Here's how the part is built. I have some questions about the finished solid (model axes, mm). A direction names the side the tool comes from. Give positions to 0.01 mm unless a question says otherwise; leave off trailing zeros. Order: outer loops, then holes, each group sorted by start corner. A loop starts at its lowest first (then second) coordinate and runs counter-clockwise, first axis right, second up.
Autodesk Inventor part; units mm, degrees
ref_plane "YZ Plane" through (0, 0, 0) normal (1, 0, 0) x (0, 1, 0)
ref_plane "XZ Plane" through (0, 0, 0) normal (0, 1, 0) x (-1, 0, 0)
ref_plane "XY Plane" through (0, 0, 0) normal (0, 0, 1) x (1, 0, 0)
sketch "Sketch1" plane through (0, 0, 0) normal (0, 1, 0) x (-1, 0, 0)
  line L0 (0, 0) -> (-20, 0)
  line L1 (-20, 0) -> (-20, -3)
  line L2 (-20, -3) -> (0, -3)
  line L3 (0, -3) -> (0, 0)
  line L4 (3, -6) -> (-23, -6)
  line L5 (-23, -6) -> (-23, 3)
  line L6 (-23, 3) -> (3, 3)
  line L7 (3, 3) -> (3, -6)
  line L8 (-30, -6) -> (-30, 3)
  line L9 (10, 3) -> (10, -6)
  line L10 (3, -6) -> (10, -6)
  line L11 (3, 3) -> (10, 3)
  line L12 (-23, 3) -> (-30, 3)
  line L13 (-23, -6) -> (-30, -6)
  line L14 (10, -6) -> (13, -6)
  line L15 (13, -6) -> (13, 3)
  line L16 (13, 3) -> (10, 3)
  line L17 (-30, 3) -> (-33, 3)
  line L18 (-33, 3) -> (-33, -6)
  line L19 (-33, -6) -> (-30, -6)
  line L20 (0, 0) -> (10, 0)
  line L21 (0, -3) -> (10, -3)
  line L22 (-20, 0) -> (-30, 0)
  line L23 (-20, -3) -> (-30, -3)
  dimension "d0" = 20
  dimension "d1" = 3
  dimension "d2" = 3
  dimension "d6" = 40
  dimension "d7" = 3
  dimension "d8" = 3
extrude "Extrusion1" add sketch "Sketch1" against normal blind 3 contours L20 L7 L21 L3 | L0 L22 L5 L6 L7 L20 | L1 L23 L5 L22 | L21 L7 L4 L5 L23 L2 | L20 L9 L21 L7 | L7 L11 L9 L20 | L22 L8 L12 L5 | L5 L23 L8 L22 | L21 L9 L10 L7 | L9 L16 L15 L14 | L5 L13 L8 L23 | L8 L19 L18 L17
extrude "Extrusion2" add sketch "Sketch1" along normal blind 40 contours L0 L22 L5 L6 L7 L20 | L21 L7 L4 L5 L23 L2 | L7 L11 L9 L20 | L22 L8 L12 L5 | L21 L9 L10 L7 | L9 L16 L15 L14 | L5 L13 L8 L23 | L8 L19 L18 L17
sketch "Sketch2" plane through (0, 40, 0) normal (0, 1, 0) x (1, 0, 0)
  line L0 (33, 6) -> (-13, 6)
  line L1 (-13, 6) -> (-13, -3)
  line L2 (-13, -3) -> (33, -3)
  line L3 (33, -3) -> (33, 6)
  line L4 (-10, 3) -> (30, 3)
  line L5 (30, 3) -> (30, 0)
  line L6 (30, 0) -> (-10, 0)
  line L7 (-10, 0) -> (-10, 3)
  point P0 (0, 0)
extrude "Extrusion3" add sketch "Sketch2" along normal blind 3 contours L3 L2 L1 L0 | L4 L5 L6 L7
sketch "Sketch3" plane through (-13, -3, 3) normal (0, 0, 1) x (1, 0, 0)
  line L0 (7, 43) -> (39, 43)
  line L1 (43, 39) -> (43, 7)
  line L2 (39, 3) -> (7, 3)
  line L3 (3, 7) -> (3, 39)
  line L4 (0, 46) -> (0, 0)
  line L5 (46, 0) -> (0, 0)
  line L6 (46, 0) -> (46, 46)
  line L7 (0, 46) -> (46, 46)
  arc A0 (7, 43) -> (3, 39) centre (7, 39) ccw
  arc A1 (43, 39) -> (39, 43) centre (39, 39) ccw
  arc A2 (39, 3) -> (43, 7) centre (39, 7) ccw
  arc A3 (3, 7) -> (7, 3) centre (7, 7) ccw
  line L8 (43, 3) -> (33, 3)
  line L9 (43, 3) -> (39, 3)
  line L10 (43, 3) -> (43, 43)
  line L11 (43, 3) -> (43, 7)
  point P0 (13, 3)
  point P1 (3, 43)
  point P2 (3, 3)
  dimension "d13" = 40
  dimension "d14" = 40
  dimension "d15" = 3
  dimension "d16" = 3
  dimension "d21" = 4
extrude "Extrusion4" cut sketch "Sketch3" against normal blind 3 contours L0 A1 L1 A2 L2 A3 L3 A0
extrude "Extrusion6" add sketch "Sketch3" against normal blind 8 contours L10 L8 A2 | L7 L6 L5 L4
extrude "Extrusion7" add sketch "Sketch3" along normal blind 10.5 contours L10 L8 A2 | L7 L6 L5 L4
extrude "Extrusion8" cut sketch "Sketch1" against normal blind 10.5 contours L3 L2 L1 L0
fillet "Fillet1" radius 5 4 edges at (-13, 43, 3.75) (33, 43, 3.75) (-13, -3, 3.75) (33, -3, 3.75)
sketch "Sketch4" plane through (-13, -3, 13.5) normal (0, 0, 1) x (1, 0, 0)
  arc A0 (41, 0) -> (46, 5) centre (41, 5) ccw
  line L0 (46, 5) -> (46, 41)
  arc A1 (46, 41) -> (41, 46) centre (41, 41) ccw
  line L1 (41, 46) -> (5, 46)
  arc A2 (5, 46) -> (0, 41) centre (5, 41) ccw
  line L2 (0, 41) -> (0, 5)
  arc A3 (0, 5) -> (5, 0) centre (5, 5) ccw
  line L3 (5, 0) -> (41, 0)
  line L4 (7, 43) -> (39, 43)
  arc A4 (43, 39) -> (39, 43) centre (39, 39) ccw
  line L5 (43, 39) -> (43, 7)
  arc A5 (39, 3) -> (43, 7) centre (39, 7) ccw
  line L6 (39, 3) -> (7, 3)
  arc A6 (3, 7) -> (7, 3) centre (7, 7) ccw
  line L7 (3, 7) -> (3, 39)
  arc A7 (7, 43) -> (3, 39) centre (7, 39) ccw
  arc A8 (0, 5) -> (5, 0) centre (5, 5) ccw
  line L8 (0, 5) -> (-2.5, 5)
  line L9 (-7.5, 10) -> (-7.5, 10)
  line L10 (-2.5, 15) -> (0, 15)
  arc A9 (-2.5, 15) -> (-7.5, 10) centre (-2.5, 10) ccw
  arc A10 (-7.5, 10) -> (-2.5, 5) centre (-2.5, 10) ccw
  line L11 (46, 5) -> (48.5, 5)
  line L12 (53.5, 10) -> (53.5, 10)
  line L13 (48.5, 15) -> (46, 15)
  line L14 (46, 15) -> (46, 5)
  circle A11 centre (48.5, 10) radius 2.5
  arc A12 (53.5, 10) -> (48.5, 15) centre (48.5, 10) ccw
  arc A13 (48.5, 5) -> (53.5, 10) centre (48.5, 10) ccw
  circle A14 centre (-2.5, 10) radius 2.5
  point P0 (13, 3)
  point P1 (-7.5, 5)
  point P2 (-7.5, 15)
  point P3 (-7.5, 10)
  point P4 (53.5, 15)
  point P5 (53.5, 5)
  point P6 (53.5, 10)
  point P7 (46, 10)
  point P8 (-7.5, 10)
  point P9 (0, 10)
  dimension "d29" = 7.5
  dimension "d30" = 10
  dimension "d33" = 5
  dimension "d34" = 7.5
  dimension "d35" = 10
  dimension "d36" = 5
  dimension "d37" = 5
  dimension "d38" = 5
  dimension "d41" = 5
extrude "Extrusion9" add sketch "Sketch4" against normal blind 10 contours L0 L13 A12 A13 L11 | L8 A10 A9 L10 L2
fillet "Fillet2" radius 2 3 edges at (-10, 20, -3) (10, 40, -3) (30, 20, -3)
fillet "Fillet4" radius 2.5 6 edges at (34.25, 2, 3.5) (34.25, 12, 3.5) (40.5, 7, 3.5) (-14.25, 12, 3.5) (-14.25, 2, 3.5) (-20.5, 7, 3.5)
properties part number "FANHOLDER_3DPrint"
Q1. If we section it at B-B on z = 10.75: List the corners of the cut face in (x, y) for me.
Filled sheet:
outline: (-15.5, 2) - (-13, 2) arc R5 ccw to (-8, -3) - (28, -3) arc R5 ccw to (33, 2) - (35.5, 2) arc R5 ccw to (35.5, 12) - (33, 12) - (33, 38) arc R5 ccw to (28, 43) - (-8, 43) arc R5 ccw to (-13, 38) - (-13, 12) - (-15.5, 12) arc R5 ccw to start; hole circle Ø5 at (-15.5, 7); hole (-10, 4) arc R4 ccw to (-6, 0) - (26, 0) arc R4 ccw to (30, 4) - (30, 36) arc R4 ccw to (26, 40) - (-6, 40) arc R4 ccw to (-10, 36) - close; hole circle Ø5 at (35.5, 7)
Q2. If we section it at A-A on x = 1: List the corners of the cut face in (y, z) for me, plus the area to 3 significant figures.
Filled sheet:
outline: (-3, -6) - (43, -6) - (43, 13.5) - (40, 13.5) - (40, -1) arc R2 cw to (38, -3) - (-3, -3) - close; (-3, 0) - (0, 0) - (0, 13.5) - (-3, 13.5) - close
area: 229 mm2
Q3. I'm going to push flat-ended pins straight in: P1, Ø11.5, axis at y = 23, z = 8.5, coming from the -X side; P2, Ø1.2, axis at x = 34.5, z = 9.5, coming from the +Y side; P3, Ø2, axis at x = 21, y = 36.5, coming from the +Z side. Where does each tip first touch, or does it pass through?
Filled sheet:
P1: stops at x = -13
P2: stops at y = 12
P3: stops at z = -3
Q4. If we section it at C-C on x = 21: List the corners of the cut face in (y, z) for me, plus the area to 3 significant figures.
Filled sheet:
outline: (-3, -6) - (43, -6) - (43, 13.5) - (40, 13.5) - (40, -1) arc R2 cw to (38, -3) - (2, -3) arc R2 cw to (0, -1) - (0, 13.5) - (-3, 13.5) - close
area: 239 mm2
Q5. For faces 4 (the face through (10, 40, 6)), 5 (the face through (-14, 12, 10)), 6 (the face through (34, 12, 10)), 7 (the face through (-20.5, 7.1, 9.8)), which set-ups out of +Z, -Z, +X, -X, +Y, -Y let a thin tool reach every point of the face, with its end or its side?
Filled sheet:
face 4: +Z
face 5: +Z, -Z, -X, +Y
face 6: +Z, -Z, +X, +Y
face 7: +Z, -Z, -X
Q6. If we section it at D-D on y = 15: List the corners of the cut face in (x, z) for me, plus the area to 3 significant figures.
Filled sheet:
outline: (-13, -6) - (33, -6) - (33, 13.5) - (30, 13.5) - (30, -1) arc R2 cw to (28, -3) - (-8, -3) arc R2 cw to (-10, -1) - (-10, 13.5) - (-13, 13.5) - close
area: 239 mm2
Q7. I need wall thicknesses on L1, parallel to X at y = 34, z = 0.75; L2, parallel to Y at x = 20, z = 9.25; L3, parallel to Y at x = 35.5, z = 6.75. Which ranges of each line are inside material? Lowest first, please.
Filled sheet:
L1: x = -13 to -10, 30 to 33
L2: y = -3 to 0, 40 to 43
L3: y = 2 to 4.5, 9.5 to 12
Q8. Thinking about a two-plate mould opening in Z: for faces 1 (the face through (31, -2, 4)), 2 (the face through (10, -1, 0)), 3 (the face through (10, 20, -6)), which applies, released by +Z, released by -Z, zero draft, split by the parting line, or undercut?
Filled sheet:
face 1: zero draft
face 2: undercut
face 3: released by -Z
